Autodesk Fusion 360 part; units mm, degrees
sketch "Sketch1" plane through (0, 0, 0) normal (0, 0, 1) x (1, 0, 0)
  line L0 (0, 0) -> (299, 0)
  line L1 (299, 0) -> (299, 135)
  line L2 (299, 135) -> (0, 135)
  line L3 (0, 135) -> (0, 0)
  line L4 (0, 135) -> (3, 135)
  line L5 (3, 130) -> (296, 130)
  line L6 (296, 130) -> (296, 5)
  line L7 (296, 5) -> (3, 5)
  line L8 (3, 5) -> (3, 130)
  dimension "d1" = 299
  dimension "d2" = 135
  dimension "d3" = 3
extrude "Extrude1" add sketch "Sketch1" along normal blind 13
sketch "Sketch2" plane through (0, 0, 0) normal (0, 0, 1) x (1, 0, 0)
  line L0 (3, 130) -> (296, 130)
  line L1 (296, 130) -> (296, 5)
  line L2 (296, 5) -> (3, 5)
  line L3 (3, 5) -> (3, 130)
extrude "Extrude2" add sketch "Sketch2" along normal blind 3
extrude "Extrude3" add 1 faces at (100.6667, 1.6667, 13) along direction (0, 0, 1) blind 5
extrude "Extrude4" add 1 faces at (100.6667, 88.3333, 3) along direction (0, 0, 1) blind 2
sketch "Sketch3" plane through (0, 0, 0) normal (-1, 0, 0) x (0, -1, 0)
  line L0 (-135, 0) -> (0, 0)
  line L1 (0, 0) -> (0, 18)
  line L2 (0, 18) -> (-135, 18)
  line L3 (-135, 18) -> (-135, 0)
  line L4 (-130, 15) -> (-100, 15)
  line L5 (-100, 15) -> (-100, 5)
  line L6 (-100, 5) -> (-130, 5)
  line L7 (-130, 5) -> (-130, 15)
  dimension "d12" = 10
extrude "Extrude5" cut sketch "Sketch3" against normal blind 10 contours L4 L5 L6 L7
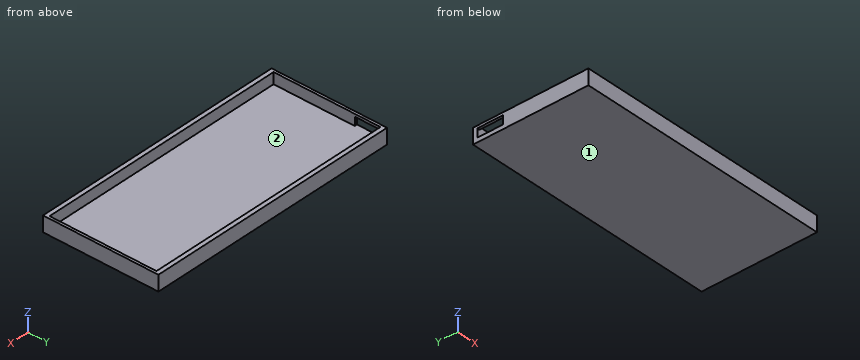
Model file for the job. Use its own axes, mm. Face numbers are marked on the shaded views. Give positions to 0.01 mm unless a question says otherwise; leave off trailing zeros. Loops run counter-clockwise (first coordinate to the right, second up) from the corner with the lowest first, then second, coordinate; pieces in that order, holes last. Notation, with made-up numbers: (-21.75, -25.75) - (6.25, -25.75) arc R24 ccw to (6.25, -3.75) - close; hole circle Ø1 at (-13.75, -20.5). An arc over 180 degrees is marked (long way). One line per item, written item: value. Start each with the question number.
1. Probe L1, parallel to Y at x = 77.5, z = 5.25; L2, parallel to X at y = 20, z = 11; L3, parallel to Z at x = 205, y = 81.5. List the from-to ranges inside material, lowest first. Write a range as from..to.
2. Slice it at B-B (x = 84.5). List the corners of the cut face in (y, z).
3. Slice it at A-A (y = 104). List the corners of the cut face in (x, z), plus the area to 3 significant figures.
4. Pin check, flat tip, straight feed: pin 1 (1.5 mm diameter, centred on x = 63, y = 77, fed in from -Z). Stop position of the tip, or through.
5. Pull direction X, two halves, no side cores. Call the marked faces 1 and 2: pulls with the +X half, pulls with the -X half, needs draft (parallel to the pull), parting line crosses it, or undercut.
6. Slice it at C-C (y = 86). List the corners of the cut face in (x, z), plus the area to 3 significant figures.
Solution:
1. L1: y = 0..5, 130..135
1. L2: x = 0..3, 296..299
1. L3: z = 0..5
2. outline: (0, 0) - (135, 0) - (135, 18) - (130, 18) - (130, 5) - (5, 5) - (5, 18) - (0, 18) - close
3. outline: (0, 0) - (299, 0) - (299, 18) - (296, 18) - (296, 5) - (0, 5) - close; (0, 15) - (3, 15) - (3, 18) - (0, 18) - close
3. area: 1,540 mm^2
4. pin 1: stops at z = 0
5. face 1: needs draft
5. face 2: undercut
6. outline: (0, 0) - (299, 0) - (299, 18) - (296, 18) - (296, 5) - (3, 5) - (3, 18) - (0, 18) - close
6. area: 1,570 mm^2
